Build history of the part. All positions in model axes, mm. Round coordinates to 2 decimals unless told otherwise and drop trailing zeros. Write each loop counter-clockwise with the first axis right and the second up, starting at its lowest first coordinate (ties: lowest second). Pieces come first, ordered by that corner, then holes.
1) Saw through at A-A (z = 28). Write the cut outline in (x, y), plus the area to 3 significant figures.
2) Wall check: probe 1 along X at (y, z) = (0.3, -10); probe 2 along X at (y, z) = (1.3, -43.5); probe 3 along X at (y, z) = (3.1, 23). Give the ranges that are in metal, low to high.
3) Saw through at B-B (z = 80). Write the cut outline in (x, y), plus the area to 3 significant figures.
4) Saw through at C-C (x = 1). Write the cut outline in (y, z).
5) Flat gauge pins, fed straight in: pin 1 (5 mm diameter, centred on x = 40, z = 62, fed in from +Y); pin 2 (3 mm diameter, centred on x = -35, y = 3, fed in from +Z); pin 3 (2.5 mm diameter, centred on x = -39, z = -65, fed in from +Y); pin 4 (1.1 mm diameter, centred on y = 5.5, z = -73, fed in from +X). Where does each tip first touch, or does it go through?
from build123d import *

# Parameters (mm, degrees)
SKETCH1_R           = 1.6
BOSS_EXTRUDE1_DEPTH = 6
FILLET1_R           = 20
CUT_EXTRUDE1_REACH  = 125.376
FILLET4_R           = 5
SKETCH6_W           = 6.4
SKETCH6_H           = 33.317887839
SKETCH6_H_2         = 25.783254567
CUT_EXTRUDE2_DEPTH  = 1
SKETCH7_R           = 3.1
CUT_EXTRUDE3_DEPTH  = 1
CHAMFER1_SIZE       = 1.5


with BuildPart() as part:
    # Sketch1 → Boss-Extrude1 (new body)
    with BuildSketch(Plane(origin=(0, 0, 0), x_dir=(1, 0, 0), z_dir=(0, 1, 0))):
        with BuildLine():
            Line((-62.882592423, 95.340725775), (0, 45))
            Line((0, 45), (62.882592423, 95.340725775))
            ThreePointArc((62.882592423, 95.340725775), (72.454956907, 95.659779271), (75.473207923, 86.570108333))
            Line((75.473207923, 86.570108333), (50, 10))
            Line((50, 10), (75.617337378, -87.053778983))
            ThreePointArc((75.617337378, -87.053778983), (71.66966075, -96.142122248), (61.911734553, -94.420201694))
            Line((61.911734553, -94.420201694), (0, -25))
            Line((0, -25), (-61.911734553, -94.420201694))
            ThreePointArc((-61.911734553, -94.420201694), (-71.66966075, -96.142122248), (-75.617337378, -87.053778983))
            Line((-75.617337378, -87.053778983), (-50, 10))
            Line((-50, 10), (-75.473207923, 86.570108333))
            ThreePointArc((-75.473207923, 86.570108333), (-72.454956907, 95.659779271), (-62.882592423, 95.340725775))
        make_face()
        with Locations(Location((-67.882250994, 89.09545443, 0), (0, 0, 270))):
            Circle(SKETCH1_R, mode=Mode.SUBTRACT)
        with Locations(Location((67.882250994, 89.09545443, 0), (0, 0, 270))):
            Circle(SKETCH1_R, mode=Mode.SUBTRACT)
        with Locations(Location((-67.882250994, -89.09545443, 0), (0, 0, 270))):
            Circle(SKETCH1_R, mode=Mode.SUBTRACT)
        with Locations(Location((67.882250994, -89.09545443, 0), (0, 0, 270))):
            Circle(SKETCH1_R, mode=Mode.SUBTRACT)
        with Locations(Location((-39, 65, 0), (0, 0, 270))):
            Circle(SKETCH1_R, mode=Mode.SUBTRACT)
        with Locations(Location((39, 65, 0), (0, 0, 270))):
            Circle(SKETCH1_R, mode=Mode.SUBTRACT)
        with Locations(Location((39, -55, 0), (0, 0, 270))):
            Circle(SKETCH1_R, mode=Mode.SUBTRACT)
        with Locations(Location((-39, -55, 0), (0, 0, 270))):
            Circle(SKETCH1_R, mode=Mode.SUBTRACT)
    extrude(amount=BOSS_EXTRUDE1_DEPTH)

    # Fillet1
    fillet1_edges = [part.edges().sort_by_distance(p)[0] for p in [
        (0, 3, -45),
        (50, 3, -10),
        (0, 3, 25),
        (-50, 3, -10),
    ]]
    fillet(fillet1_edges, radius=FILLET1_R)

    # Sketch2 → Cut-Extrude1 (cut, up to next)
    with BuildSketch(Plane(origin=(0, 6, 0), x_dir=(1, 0, 0), z_dir=(0, 1, 0)), mode=Mode.PRIVATE) as cut_extrude1_sk1:
        with BuildLine():
            Line((-53.761195119, 68.824044103), (-37.648281191, 20.390114276))
            ThreePointArc((-37.648281191, 20.390114276), (-35.876133945, 10.445731448), (-37.017714824, 0.409395025))
            Line((-37.017714824, 0.409395025), (-53.656219744, -62.627202233))
            Line((-53.656219744, -62.627202233), (-26.12100943, -31.752605236))
            ThreePointArc((-26.12100943, -31.752605236), (0, -20.048374517), (26.12100943, -31.752605236))
            Line((26.12100943, -31.752605236), (53.656219744, -62.627202233))
            Line((53.656219744, -62.627202233), (37.017714824, 0.409395025))
            ThreePointArc((37.017714824, 0.409395025), (35.876133945, 10.445731448), (37.648281191, 20.390114276))
            Line((37.648281191, 20.390114276), (53.761195119, 68.824044103))
            Line((53.761195119, 68.824044103), (21.873506248, 43.296321101))
            ThreePointArc((21.873506248, 43.296321101), (0, 35.619383236), (-21.873506248, 43.296321101))
            Line((-21.873506248, 43.296321101), (-53.761195119, 68.824044103))
        make_face()
    cut_extrude1_tool1 = extrude(cut_extrude1_sk1.sketch, amount=-CUT_EXTRUDE1_REACH, mode=Mode.PRIVATE) & part.part
    add(cut_extrude1_tool1.solids().sort_by_distance((0, 6, -6.295596))[0], mode=Mode.SUBTRACT)

    # Fillet4
    fillet4_edges = [part.edges().sort_by_distance(p)[0] for p in [
        (-53.761195119, 3, -68.824044103),
        (53.761195119, 3, -68.824044103),
        (53.656219744, 3, 62.627202233),
        (-53.656219744, 3, 62.627202233),
    ]]
    fillet(fillet4_edges, radius=FILLET4_R)

    # Sketch6 → Cut-Extrude2 (cut)
    with BuildSketch(Plane(origin=(0, 6, 0), x_dir=(1, 0, 0), z_dir=(0, 1, 0))):
        with Locations((-39, -55.65894392)):
            Rectangle(SKETCH6_W, SKETCH6_H)
        with Locations((39, -55.65894392)):
            Rectangle(SKETCH6_W, SKETCH6_H)
        with Locations((39, 65.891627284)):
            Rectangle(SKETCH6_W, SKETCH6_H_2)
        with Locations((-39, 65.891627284)):
            Rectangle(SKETCH6_W, SKETCH6_H_2)
    extrude(amount=-CUT_EXTRUDE2_DEPTH, mode=Mode.SUBTRACT)

    # Sketch7 → Cut-Extrude3 (cut)
    with BuildSketch(Plane.XZ):
        with Locations(Location((-39, 55, 0), (0, 0, 270))):
            Circle(SKETCH7_R)
        with Locations(Location((39, 55, 0), (0, 0, 270))):
            Circle(SKETCH7_R)
        with Locations(Location((-39, -65, 0), (0, 0, 270))):
            Circle(SKETCH7_R)
        with Locations(Location((39, -65, 0), (0, 0, 270))):
            Circle(SKETCH7_R)
    extrude(amount=-CUT_EXTRUDE3_DEPTH, mode=Mode.SUBTRACT)

    # Chamfer1
    chamfer1_edges = [part.edges().sort_by_distance(p)[0] for p in [
        (-39, 1, 53.4),
        (39, 1, 53.4),
        (-39, 1, -66.6),
        (39, 1, -66.6),
    ]]
    chamfer(chamfer1_edges, length=CHAMFER1_SIZE - 0.0001)  # a hair under: the kernel refuses the full size


solid = part.part
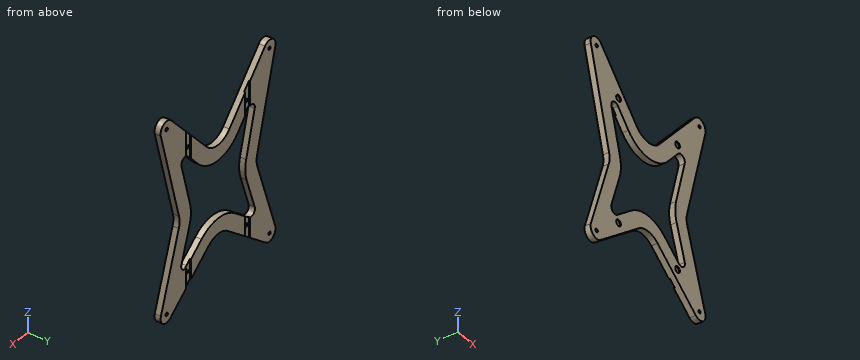
Evaluation:
1. outline: (-60.03, 0) - (-44.52, 0) - (-44.52, 6) - (-60.03, 6) - close; (-22.21, 0) - (22.21, 0) - (22.21, 6) - (-22.21, 6) - close; (44.52, 0) - (60.03, 0) - (60.03, 6) - (44.52, 6) - close
1. area: 453 mm2
2. probe 1: x = -50.87 to -35.86, 35.86 to 50.87
2. probe 2: x = -61.14 to -45.34, -22.13 to 22.13, 45.34 to 61.14
2. probe 3: x = -58.71 to -43.2, -14.07 to 14.07, 43.2 to 58.71
3. outline: (-73.76, 0) - (-49.05, 0) - (-49.05, 6) - (-73.76, 6) - close; (49.05, 0) - (73.76, 0) - (73.76, 6) - (49.05, 6) - close
3. area: 296 mm2
4. outline: (0, -50.64) - (6, -50.64) - (6, -35.63) - (0, -35.63) - close; (0, 20.06) - (6, 20.06) - (6, 35.07) - (0, 35.07) - close
5. pin 1: stops at y = 6
5. pin 2: stops at z = 65.93
5. pin 3: passes through
5. pin 4: stops at x = 71.14
